CAD build for the part. Positions are in the model's coordinates, mm. A direction names the side the tool comes from. Round coordinates to 2 decimals unless told otherwise and drop trailing zeros. Loops run counter-clockwise (first coordinate to the right, second up) from the corner with the lowest first, then second, coordinate; pieces in that order, holes last. Notation, with made-up numbers: M 34,54 L 60,54 A21 ccw 60,59 Z; hole C -31.75,9.5 d1. An arc over 180 degrees is marked long. Use a Markdown table: item, result. Add a question column.
(1) Wall check: L1, parallel to X at y = 0.85, z = -50; L2, parallel to X at y = 2.35, z = -30. Give the ranges that are in metal, low to high.
(2) Band-saw the part on A-A, the plane x = -10. Write the cut outline in (y, z), and give its area (3 significant figures).
(3) Band-saw the part on D-D, the plane y = 0.6. Give the number of separate pieces and of enclosed holes in the cut face, and give its area (3 significant figures).
(4) Band-saw the part on B-B, the plane z = -10. Write the cut outline in (x, y).
(5) Two-plate mould, pull along X, no slides. Class faces 1 (the face through (-72.4, 1.5, -68.2)), 2 (the face through (0, 1, -40)), 3 (the face through (-80, 1, -60)), 4 (the face through (-10, 2, -53)): released by +X, released by -X, zero draft, split by the parting line, or undercut.
(6) Which spindle directions (+Z, -Z, +X, -X, +Y, -Y) get a long thin tool onto all of the face, cutting with end or side? Do faces 5 (the face through (-72.21, 1.52, -52.03)), 6 (the face through (-40, 1, -20)). Say none if no direction does.
(7) Band-saw the part on C-C, the plane z = -70. Write the cut outline in (x, y).
(8) Flat gauge pins, fed straight in: P1, Ø9.5, axis at x = -70, z = -70, coming from the +Y side; P2, Ø1.5, axis at x = -48, y = 2.5, coming from the +Z side. Where does each tip first touch, or does it go through?
Autodesk Inventor part; units mm, degrees
ref_plane "YZ Plane" through (0, 0, 0) normal (1, 0, 0) x (0, 1, 0)
ref_plane "XZ Plane" through (0, 0, 0) normal (0, 1, 0) x (-1, 0, 0)
ref_plane "XY Plane" through (0, 0, 0) normal (0, 0, 1) x (1, 0, 0)
sketch "Sketch1" plane through (0, 0, 0) normal (0, 1, 0) x (-1, 0, 0)
  line L0 (0, 0) -> (40, 0)
  line L1 (40, 0) -> (40, -80)
  line L2 (40, -80) -> (0, -80)
  line L3 (0, -80) -> (0, 0)
  line L4 (0, -80) -> (80, -80)
  line L5 (80, -80) -> (80, -40)
  line L6 (80, -40) -> (0, -40)
  line L7 (0, -40) -> (0, -80)
  point P0 (40, -40)
  dimension "d0" = 40
  dimension "d1" = 80
  dimension "d2" = 80
  dimension "d3" = 40
extrude "Extrusion1" add sketch "Sketch1" along normal blind 3
sketch "Sketch2" plane through (0, 3, 0) normal (0, 1, 0) x (1, 0, 0)
  line L0 (0, 0) -> (-10, 0)
  line L1 (-40, 0) -> (0, 0)
  line L2 (-10, 0) -> (-10, 10)
  circle A0 centre (-10, 10) radius 3
  line L3 (0, 0) -> (0, 80)
  line L4 (0, 0) -> (0, 80)
  circle A1 centre (-10, 30) radius 3
  circle A2 centre (-10, 50) radius 3
  circle A3 centre (-10, 70) radius 3
  circle A4 centre (-30, 10) radius 3
  circle A5 centre (-30, 30) radius 3
  circle A6 centre (-30, 50) radius 3
  circle A7 centre (-30, 70) radius 3
  line L5 (-10, 70) -> (0, 70)
  line L6 (-10, 70) -> (-10, 80)
  line L7 (0, 80) -> (-80, 80)
  circle A8 centre (-10, 70) radius 3
  circle A9 centre (-30, 70) radius 3
  circle A10 centre (-50, 70) radius 3
  circle A11 centre (-70, 70) radius 3
  circle A12 centre (-10, 50) radius 3
  circle A13 centre (-30, 50) radius 3
  circle A14 centre (-50, 50) radius 3
  circle A15 centre (-70, 50) radius 3
  dimension "d6" = 10
  dimension "d7" = 10
  dimension "d8" = 6
  dimension "d11" = 20
  dimension "d14" = 20
  dimension "d19" = 20
  dimension "d22" = 20
extrude "Extrusion2" cut sketch "Sketch2" against normal through all contours A0 | L5 L6 A3 | A3 L6 L5 | A1 | A2 | A4 | A5 | A6 | A7 | A10 | A11 | A14 | A15
fillet "Fillet1" radius 5 6 edges at (0, 1.5, 0) (-40, 1.5, 0) (0, 1.5, -80) (-40, 1.5, -40) (-80, 1.5, -40) (-80, 1.5, -80)
properties part number "RightAngle_4040"
Return value:
| question | item | result |
|---|---|---|
| 1 | L1 | -80 to -73, -67 to -53, -47 to -33, -27 to -13, -7 to 0 |
| 1 | L2 | -40 to -33, -27 to -13, -7 to 0 |
| 2 | outline | M 0,-80 L 3,-80 L 3,-73 L 0,-73 Z; M 0,-67 L 3,-67 L 3,-53 L 0,-53 Z; M 0,-47 L 3,-47 L 3,-33 L 0,-33 Z; M 0,-27 L 3,-27 L 3,-13 L 0,-13 Z; M 0,-7 L 3,-7 L 3,0 L 0,0 Z |
| 2 | area | 168 mm^2 |
| 3 | separate pieces | 1 |
| 3 | enclosed holes | 12 |
| 3 | area | 4,440 mm^2 |
| 4 | outline | M -40,0 L -33,0 L -33,3 L -40,3 Z; M -27,0 L -13,0 L -13,3 L -27,3 Z; M -7,0 L 0,0 L 0,3 L -7,3 Z |
| 5 | face 1 | undercut |
| 5 | face 2 | released by +X |
| 5 | face 3 | released by -X |
| 5 | face 4 | undercut |
| 6 | face 5 | +Y, -Y |
| 6 | face 6 | +Z, -X, +Y, -Y |
| 7 | outline | M -80,0 L -73,0 L -73,3 L -80,3 Z; M -67,0 L -53,0 L -53,3 L -67,3 Z; M -47,0 L -33,0 L -33,3 L -47,3 Z; M -27,0 L -13,0 L -13,3 L -27,3 Z; M -7,0 L 0,0 L 0,3 L -7,3 Z |
| 8 | P1 | y = 3 |
| 8 | P2 | z = -40 |
